Solid Edge part; units mm, degrees
sketch "Sketch1" plane through (0, 0, 0) normal (1, 0, 0) x (0, 1, 0)
  line L0 (-9, 115) -> (9, 115)
  line L1 (9, 115) -> (9, 0)
  line L2 (9, 0) -> (14, 0)
  line L3 (14, 0) -> (14, 120)
  line L4 (14, 120) -> (-14, 120)
  line L5 (-14, 120) -> (-14, 0)
  line L6 (-14, 0) -> (-9, 0)
  line L7 (-9, 0) -> (-9, 115)
extrude "Protrusion1" add sketch "Sketch1" along normal mid plane 40
sketch "Sketch2" plane through (0, 14, 45) normal (0, 1, 0) x (-1, 0, 0)
  line L0 (-10.1, 4) -> (-10.1, 45)
  line L1 (-10.1, 45) -> (10.1, 45)
  line L2 (10.1, 45) -> (10.1, 4)
  line L3 (10.1, 4) -> (-10.1, 4)
extrude "Cutout1" cut sketch "Sketch2" against normal up to vertex (5 mm away)
sketch "Sketch3" plane through (0, -14, 45) normal (0, -1, 0) x (1, 0, 0)
  circle A0 centre (0, 14.5) radius 12.5
extrude "Cutout2" cut sketch "Sketch3" against normal up to vertex (5 mm away)
hole "Agujero_1" at (0, -14, 21.5) direction (0, 1, 0) diameter 3.2 end through all
hole "Hole1" at (0, -14, 10.2) direction (0, 1, 0) diameter 3.2 end through all
hole "Agujero_3" at (-10, 14, 20) direction (0, -1, 0) diameter 3.2 end up to next
hole "Hole2" at (10, 14, 20) direction (0, -1, 0) diameter 3.2 end up to next
hole "Agujero_5" at (-10, 14, 110) direction (0, -1, 0) diameter 3.2 end up to next
hole "Hole3" at (10, 14, 110) direction (0, -1, 0) diameter 3.2 end up to next
sketch "Sketch4" plane through (0, 14, 60) normal (0, 1, 0) x (-1, 0, 0)
  line L0 (20, -55) -> (10, -55)
  line L1 (10, -55) -> (10, -60)
  line L2 (10, -60) -> (20, -60)
  line L3 (20, -60) -> (20, -55)
extrude "Cutout3" cut sketch "Sketch4" against normal up to vertex (5 mm away)
mirror "Mirror1" about plane through (0, 0, 0) normal (1, 0, 0) of "Cutout3"
sketch "Sketch5" plane through (0, 0, 120) normal (0, 0, 1) x (0, 1, 0)
  line L0 (-9, 20) -> (-9, 10)
  line L1 (-9, 10) -> (-14, 10)
  line L2 (-14, -10) -> (-14, 10)
  line L3 (-14, -10) -> (-9, -10)
  line L4 (-9, -10) -> (-9, -20)
  line L5 (9, -20) -> (-9, -20)
  line L6 (9, -20) -> (9, -10)
  line L7 (9, -10) -> (14, -10)
  line L8 (14, 10) -> (14, -10)
  line L9 (14, 10) -> (9, 10)
  line L10 (9, 10) -> (9, 20)
  line L11 (-9, 20) -> (9, 20)
extrude "Cutout5" cut sketch "Sketch5" against normal up to vertex (5 mm away)
sketch "Sketch6" plane through (0, 0, 120) normal (0, 0, 1) x (0, 1, 0)
  line L0 (-9, 20) -> (9, 20)
  line L1 (9, 10) -> (9, 20)
  line L2 (14, 10) -> (9, 10)
  line L3 (14, 10) -> (14, -10)
  line L4 (9, -10) -> (14, -10)
  line L5 (9, -20) -> (9, -10)
  line L6 (9, -20) -> (-9, -20)
  line L7 (-9, -10) -> (-9, -20)
  line L8 (-14, -10) -> (-9, -10)
  line L9 (-14, -10) -> (-14, 10)
  line L10 (-9, 10) -> (-14, 10)
  line L11 (-9, 20) -> (-9, 10)
extrude "Protrusion2" add sketch "Sketch6" against normal up to vertex (5 mm away)
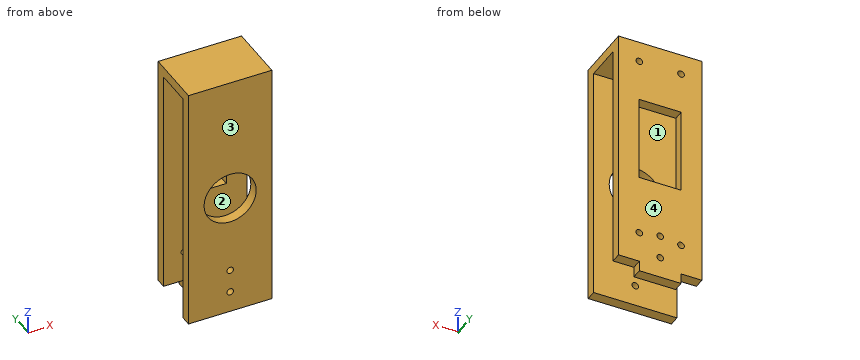
Read the model definition and answer for the solid it produces. Units are mm, in the model's axes. Face numbers are marked on the shaded views. Coordinates: 2 decimals unless noted, no trailing zeros. Loops run counter-clockwise (first coordinate to the right, second up) from the corner with the lowest first, then second, coordinate; pieces in that order, holes last. Notation, with made-up numbers: (87, 33.25) - (107, 33.25) arc R4 ccw to (107, 39.25) - close; hole circle Ø10 at (32.5, 74). An arc over 180 degrees is marked (long way). Answer in a Markdown table with one row per item.
Q1. Given P1, Ø8, axis at x = -3, y = 4.5, coming from the -Z side; P2, Ø1.5, axis at y = 10.5, z = 3, coming from the -X side; P3, Ø2.5, axis at x = -15, y = 12, coming from the -Z side, each flat-ended and moving along its own axis, determine where each tip first touches the part or whether it passes through.
Here are the results:
| item | result |
|---|---|
| P1 | stops at z = 115 |
| P2 | stops at x = -10 |
| P3 | stops at z = 5 |
Q2. The mould has two halves that part along Y. Classify the marked faces 1, 2, 3 and 4: pulls with the +Y half, pulls with the -Y half, needs draft (parallel to the pull), parting line crosses it, or undercut.
Here are the results:
| item | result |
|---|---|
| face 1 | undercut |
| face 2 | undercut |
| face 3 | pulls with the -Y half |
| face 4 | pulls with the +Y half |
Q3. Straight lines are drawn through the part: line 1 along X through (y, z) = (11.2, 110); line 2 along Z through (x, y) = (0, -10.55); line 3 along Y through (x, z) = (-14.5, 72.5). For each, find the intervals that lie inside material, in ascending order. Write a range as [from, to].
Here are the results:
| item | result |
|---|---|
| line 1 | x = [-20, -11.6], [-8.4, 8.4], [11.6, 20] |
| line 2 | z = [0, 8.6], [11.8, 19.9], [23.1, 47], [72, 120] |
| line 3 | y = [-14, -9], [9, 14] |
Q4. Find section D-D on y = 2.75. Write down the section's boundary in (x, z), plus the area to 3 significant figures.
Here are the results:
| item | result |
|---|---|
| outline | (-20, 115) - (20, 115) - (20, 120) - (-20, 120) - close |
| area | 200 mm^2 |
Q5. Find section C-C on x = 6.5. Write down the section's boundary in (y, z).
Here are the results:
| item | result |
|---|---|
| outline | (-14, 0) - (-9, 0) - (-9, 48.82) - (-14, 48.82) - close; (-14, 70.18) - (-9, 70.18) - (-9, 115) - (9, 115) - (9, 90) - (14, 90) - (14, 120) - (-14, 120) - close; (9, 0) - (14, 0) - (14, 49) - (9, 49) - close |
Q6. Find section B-B on z = 10.2. Write down the section's boundary in (x, y), plus the area to 3 significant figures.
Here are the results:
| item | result |
|---|---|
| outline | (-20, -14) - (-1.6, -14) - (-1.6, -9) - (-20, -9) - close; (-20, 9) - (-1.6, 9) - (-1.6, 14) - (-20, 14) - close; (1.6, -14) - (20, -14) - (20, -9) - (1.6, -9) - close; (1.6, 9) - (20, 9) - (20, 14) - (1.6, 14) - close |
| area | 368 mm^2 |
Q7. Find section A-A on x = 0. Count the separate pieces of the cut face and the enclosed holes in it, plus the area to 3 significant figures.
Here are the results:
| item | result |
|---|---|
| separate pieces | 7 |
| enclosed holes | 0 |
| area | 896 mm^2 |
